Source: three-view drawing plus pictorial views. Frame: mm from the lowest corner of the part. A direction names the side the tool comes from. Round coordinates to 2 decimals unless told otherwise and drop trailing zeros. Loops run counter-clockwise (first coordinate to the right, second up) from the corner with the lowest first, then second, coordinate; pieces in that order, holes last. Notation, with made-up numbers: M 29.5,60 L 44.5,60 A22 cw 44.5,84 Z; hole C 71.25,-21.75 d7. An arc over 180 degrees is marked long. Answer as a JSON object with one key per item and string values.
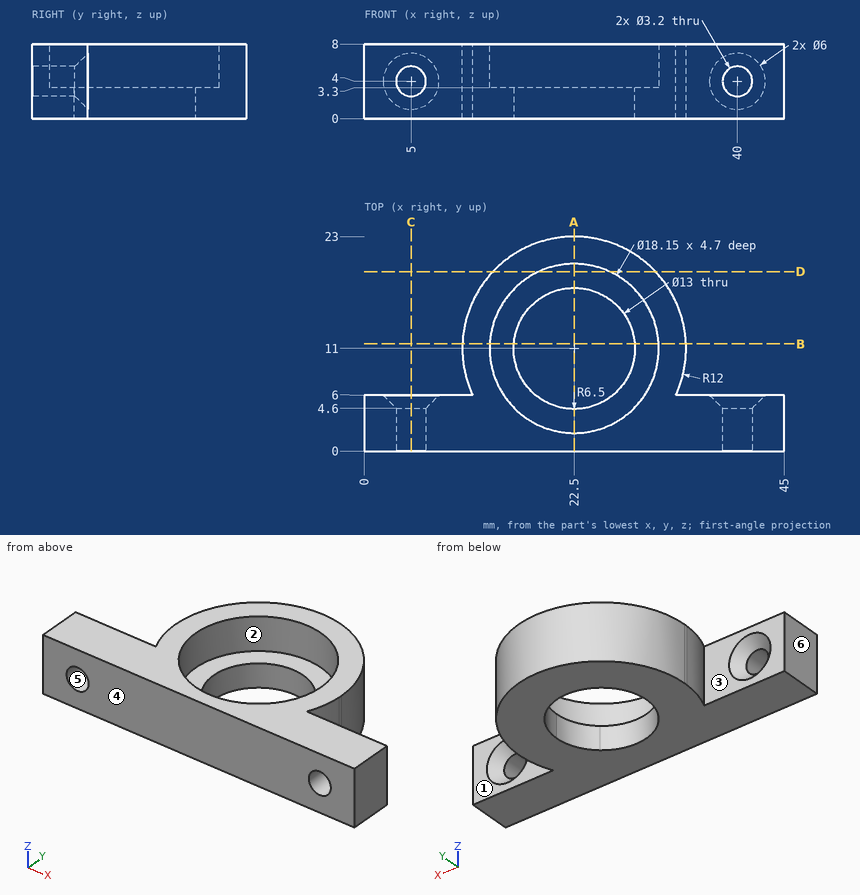
1) Line query: probe 1 along X at (y, z) = (1.85, 4); probe 2 along Z at (x, y) = (40, 1.1); probe 3 along Y at (x, z) = (22.5, 5.1) (3 decimals). Output: solid intervals per line, ascending.
Geometry results:
{"probe 1": "0 to 3.4, 6.6 to 38.4, 41.6 to 45", "probe 2": "0 to 2.4, 5.6 to 8", "probe 3": "0 to 1.925, 20.075 to 23"}
2) Set-up query: the marked faces 1, 2 and 3. Return all of +Z, -Z, +X, -X, +Y, -Y with unobstructed straight access to the full face (end or side cutting, diameter ignored); none if empty.
Geometry results:
{"face 1": "+Z, -Z, +X", "face 2": "+Z", "face 3": "+Z, -Z, -X"}
3) Pull-direction query (X, two-part tool) for the marked faces 4, 5 and 6; classes: +X half, -X half, draft (parallel to the pull), parting line (faces both ways), or undercut.
Geometry results:
{"face 4": "draft", "face 5": "undercut", "face 6": "-X half"}
4) Cut plane A-A on x = 22.5. Return the cut outline in (y, z) (3 decimals), and give its area (3 significant figures).
Geometry results:
{"outline": "M 0,0 L 4.5,0 L 4.5,3.3 L 1.925,3.3 L 1.925,8 L 0,8 Z; M 17.5,0 L 23,0 L 23,8 L 20.075,8 L 20.075,3.3 L 17.5,3.3 Z", "area": "55.8 mm2"}
5) Cut plane B-B on y = 11.5. Return the cut outline in (x, z).
Geometry results:
{"outline": "M 10.51,0 L 16.02,0 L 16.02,3.3 L 13.44,3.3 L 13.44,8 L 10.51,8 Z; M 28.98,0 L 34.49,0 L 34.49,8 L 31.56,8 L 31.56,3.3 L 28.98,3.3 Z"}
6) First-contact query: pin 1 (1 mm diameter, centred on x = 38.5, z = 6.5, fed in from +Y). Flat tip, straight axial feed; report the tip coordinate or a pass-through.
Geometry results:
{"pin 1": "y = 6"}
7) Cut plane C-C on x = 5. Return the cut outline in (y, z).
Geometry results:
{"outline": "M 0,0 L 6,0 L 6,1 L 4.6,2.4 L 0,2.4 Z; M 0,5.6 L 4.6,5.6 L 6,7 L 6,8 L 0,8 Z"}
8) Cut plane D-D on y = 19.25. Return the cut outline in (x, z), and give its area (3 significant figures).
Geometry results:
{"outline": "M 13.79,0 L 31.21,0 L 31.21,8 L 26.28,8 L 26.28,3.3 L 18.72,3.3 L 18.72,8 L 13.79,8 Z", "area": "104 mm2"}
